Print and shaded views of the part. All mm, measured from the part's lowest x, y and z. Round coordinates to 2 decimals unless told otherwise and drop trailing zeros. Write item = value, one per line.
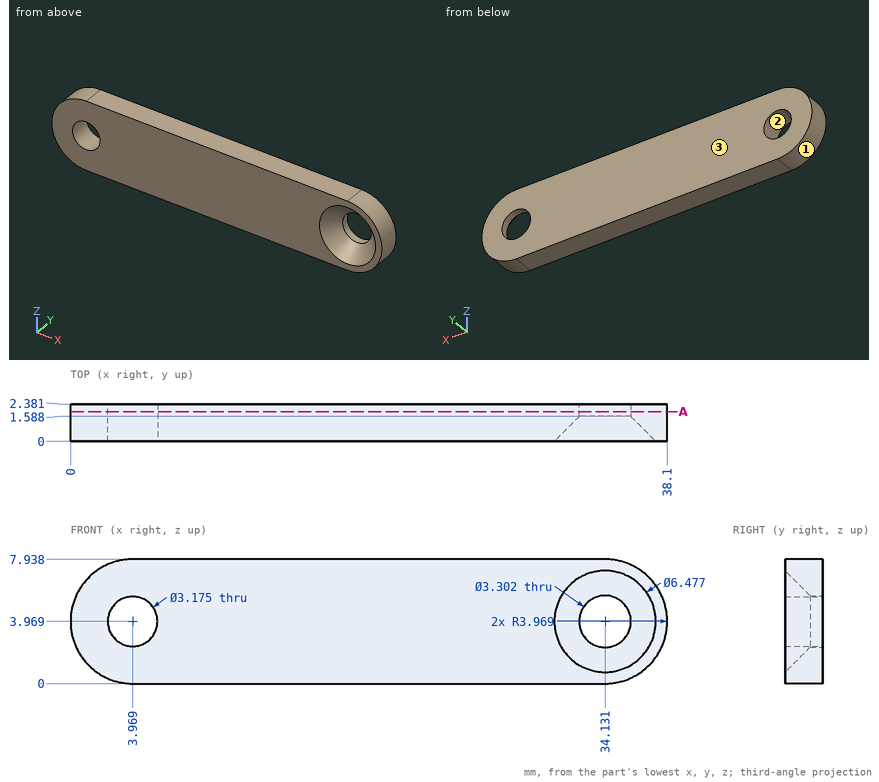
(1) Drop flat-ended pins along their axis: pin 1 (1 mm diameter, centred on x = 14, y = 1.5, fed in from -Z); pin 2 (2.5 mm diameter, centred on x = 34.13, z = 3.97, fed in from +Y). Give the stop position or say it passes through.
Solved:
pin_1 = 0
pin_2 = through
(2) Pull direction X, two halves, no side cores. Call the marked faces 1, 2 and 3: released by +X, released by -X, zero draft, split by the parting line, or undercut.
Solved:
face_1 = released by -X
face_2 = undercut
face_3 = zero draft
(3) Probe line 1 along X through (y, z) = (0.85, 5) (1 decimal); line 2 along X through (y, z) = (1.3, 3.75) (1 decimal); line 3 along Z through (x, y) = (3, 1.75) (1 decimal). List the from-to ranges inside material, lowest first.
Solved:
line_1 = 0.1 to 2.8, 5.2 to 32, 36.3 to 38
line_2 = 0 to 2.4, 5.5 to 32.2, 36.1 to 38.1
line_3 = 0.1 to 2.7, 5.2 to 7.8
(4) Band-saw the part on A-A on y = 1.9. Count the separate pieces of the cut face and the enclosed holes in it.
Solved:
separate_pieces = 1
enclosed_holes = 2
